Autodesk Inventor part; units mm, degrees
ref_plane "YZ Plane" through (0, 0, 0) normal (1, 0, 0) x (0, 1, 0)
ref_plane "XZ Plane" through (0, 0, 0) normal (0, 1, 0) x (-1, 0, 0)
ref_plane "XY Plane" through (0, 0, 0) normal (0, 0, 1) x (1, 0, 0)
sketch "Sketch1" plane through (0, 0, 0) normal (0, 0, 1) x (1, 0, 0)
  line L0 (0, 0) -> (39, 0)
  line L1 (39, 0) -> (39, 24)
  line L2 (39, 24) -> (0, 24)
  line L3 (0, 24) -> (0, 0)
  line L4 (-8.5, 24) -> (47.5, 24)
  line L5 (47.5, 24) -> (47.5, 31)
  line L6 (47.5, 31) -> (-8.5, 31)
  line L7 (-8.5, 31) -> (-8.5, 24)
  point P0 (19.5, 24)
  dimension "d0" = 39
  dimension "d1" = 24
  dimension "d2" = 56
  dimension "d3" = 7
extrude "Extrusion1" add sketch "Sketch1" along normal blind 19
sketch "Sketch2" plane through (-8.5, 31, 0) normal (0, 1, 0) x (1, 0, 0)
  circle A0 centre (18, -9.5) radius 6
  line L0 (0, 0) -> (0, -19)
  circle A1 centre (18, -9.5) radius 1.5
  point P0 (8.5, 0)
  point P1 (0, -9.5)
  dimension "d6" = 12
  dimension "d7" = 18
  dimension "d8" = 3
extrude "Extrusion2" add sketch "Sketch2" along normal blind 6
sketch "Sketch3" plane through (-8.5, 31, 0) normal (0, 1, 0) x (1, 0, 0)
  line L0 (4, -4.5) -> (52, -4.5) construction
  line L1 (52, -4.5) -> (52, -14.5) construction
  line L2 (52, -14.5) -> (4, -14.5) construction
  line L3 (4, -14.5) -> (4, -4.5) construction
  circle A0 centre (4, -4.5) radius 1.5
  circle A1 centre (4, -14.5) radius 1.5
  circle A2 centre (52, -14.5) radius 1.5
  circle A3 centre (52, -4.5) radius 1.5
  line L4 (0, 0) -> (0, -19)
  line L5 (56, 0) -> (56, -19)
  point P0 (8.5, 0)
  dimension "d11" = 3
  dimension "d12" = 3
  dimension "d13" = 3
  dimension "d14" = 3
  dimension "d15" = 4
  dimension "d16" = 4
  dimension "d17" = 4.5
  dimension "d18" = 4.5
extrude "Extrusion3" cut sketch "Sketch3" against normal blind 10
properties part number "servo"
Part model, mm, in its own coordinate system. A direction names the side the tool comes from. Coordinates: 2 decimals unless noted, no trailing zeros. Loops run counter-clockwise (first coordinate to the right, second up) from the corner with the lowest first, then second, coordinate; pieces in that order, holes last. Notation, with made-up numbers: M 33.25,37 L 37.25,37 A24 cw 37.25,61 Z; hole C 48.5,46.5 d10. An arc over 180 degrees is marked long. Use a Markdown table: item, result. Add a question column.
Q1. Cut at A-A (x = 43.5). Write the cut outline in (y, z).
Q2. Probe L1, parallel to Z at x = 43.5, y = 29.5; L2, parallel to X at y = 34.8, z = 9.5; L3, parallel to Z at x = -4, y = 26. List the from-to ranges inside material, lowest first.
Q3. Cut at C-C (z = 4.5). Write the cut outline in (x, y).
Q4. Which spindle directions (+Z, -Z, +X, -X, +Y, -Y) get a long thin tool onto all of the face, cutting with end or side? Do faces 4 (the flat face through (-4, 24, 9)), 5 (the cylindrical face through (8.3, 34, 8.6)), 6 (the flat face through (43, 24, 9)). Say none if no direction does.
Q5. Mould opens along Z. For faces 1 (the cylindrical face through (42, 27.55, 4.43)), 2 (the flat face through (11, 37, 11)), 3 (the flat face through (19, 16, 0)) say: +Z half, -Z half, draft (parallel to the pull), parting line (faces both ways), or undercut.
Q6. Pin check, flat tips, straight feed: P1, Ø3.5, axis at x = 9.5, z = 10, coming from the +Y side; P2, Ø3.5, axis at x = 43.5, z = 14.5, coming from the -Y side; P3, Ø5.5, axis at x = 32.5, z = 11, coming from the +Y side; P4, Ø3, axis at y = 20, z = 3, coming from the -X side. Stop position of each tip, or through.
Q7. Cut at D-D (y = 32.5). Write the cut outline in (x, z).
Q8. Cut at B-B (y = 27). Write the cut outline in (x, z), and give its area (3 significant figures).
Worked out:
| question | item | result |
|---|---|---|
| 1 | outline | M 24,0 L 31,0 L 31,3 L 24,3 Z; M 24,6 L 31,6 L 31,13 L 24,13 Z; M 24,16 L 31,16 L 31,19 L 24,19 Z |
| 2 | L1 | z = 0 to 3, 6 to 13, 16 to 19 |
| 2 | L2 | x = 3.5 to 8, 11 to 15.5 |
| 2 | L3 | z = 0 to 3.09, 5.91 to 13.09, 15.91 to 19 |
| 3 | outline | M -8.5,24 L -6,24 L -6,31 L -8.5,31 Z; M -3,24 L 0,24 L 0,0 L 39,0 L 39,24 L 42,24 L 42,31 L 12.82,31 L 12.82,37 L 6.18,37 L 6.18,31 L -3,31 Z; M 45,24 L 47.5,24 L 47.5,31 L 45,31 Z |
| 4 | face 4 | +Z, -Z, -X, -Y |
| 4 | face 5 | +Y |
| 4 | face 6 | +Z, -Z, +X, -Y |
| 5 | face 1 | undercut |
| 5 | face 2 | draft |
| 5 | face 3 | -Z half |
| 6 | P1 | stops at y = 37 |
| 6 | P2 | stops at y = 24 |
| 6 | P3 | stops at y = 31 |
| 6 | P4 | stops at x = 0 |
| 7 | outline | C 9.5,9.5 d12; hole C 9.5,9.5 d3 |
| 8 | outline | M -8.5,0 L 47.5,0 L 47.5,19 L -8.5,19 Z; hole C -4.5,4.5 d3; hole C -4.5,14.5 d3; hole C 43.5,4.5 d3; hole C 43.5,14.5 d3 |
| 8 | area | 1,040 mm2 |
